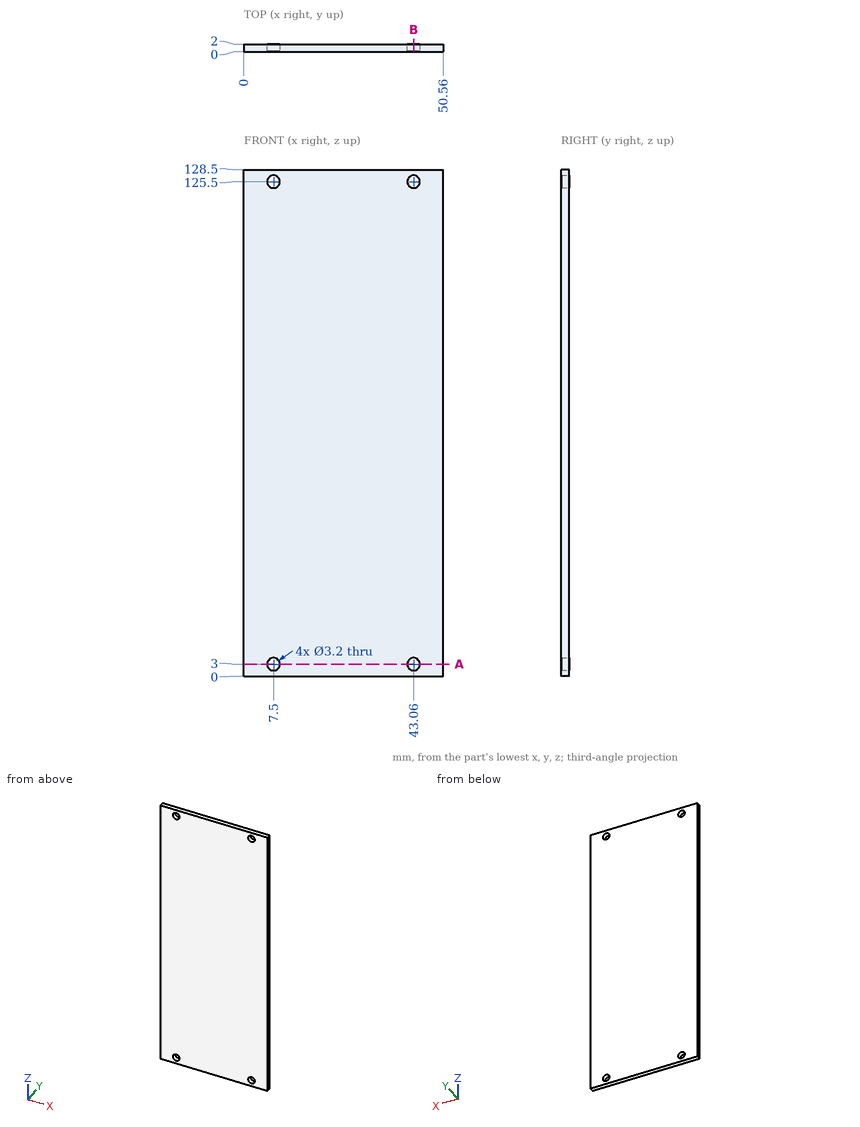
Geometry check sheet. Reference: drawing and pictorial views, mm from the part's lowest x, y, z. Coordinates: 2 decimals unless noted, no trailing zeros. Order: outer loops, then holes, each group sorted by start corner. A loop starts at its lowest first (then second) coordinate and runs counter-clockwise, first axis right, second up. Notation, with made-up numbers: (85.25, 23) -> (137.25, 23) arc R16 cw to (137.25, 51) -> close; hole circle Ø7 at (8.5, 76). An arc over 180 degrees is marked (long way). Write item = value, one per line. Start each with the question number.
1) Cross-section at B-B (x = 43.06). Enter the section's corners in (y, z).
2) Cross-section at A-A (z = 3). Enter the section's corners in (x, y), then the cut area to 3 significant figures.
3) Material ranges on L1, parallel to Z at x = 43.06, y = 0.9; L2, parallel to X at y = 0.95, z = 125.5; L3, parallel to Z at x = 7, y = 1.85, recorded low to high.
Ans:
q1.outline = (0, 0) -> (2, 0) -> (2, 1.4) -> (0, 1.4) -> close; (0, 4.6) -> (2, 4.6) -> (2, 123.9) -> (0, 123.9) -> close; (0, 127.1) -> (2, 127.1) -> (2, 128.5) -> (0, 128.5) -> close
q2.outline = (0, 0) -> (5.9, 0) -> (5.9, 2) -> (0, 2) -> close; (9.1, 0) -> (41.46, 0) -> (41.46, 2) -> (9.1, 2) -> close; (44.66, 0) -> (50.56, 0) -> (50.56, 2) -> (44.66, 2) -> close
q2.area = 88.3 mm²
q3.L1 = 0 to 1.4, 4.6 to 123.9, 127.1 to 128.5
q3.L2 = 0 to 5.9, 9.1 to 41.46, 44.66 to 50.56
q3.L3 = 0 to 1.48, 4.52 to 123.98, 127.02 to 128.5
